```python
from build123d import *

# Parameters (mm, degrees)
SKETCH1_W                  = 37.6666666
SKETCH1_H                  = 45
BOSS_EXTRUDE1_DEPTH        = 12.8
SKETCH2_W                  = 10
SKETCH2_H                  = 34
CUT_EXTRUDE1_DEPTH         = 61.063447893
CUT_EXTRUDE2_DEPTH         = 6.4
CUT_EXTRUDE3_DEPTH         = 61.063447893
CUT_EXTRUDE4_DEPTH         = 6.4
CUT_EXTRUDE5_DEPTH         = 61.063447893
F_2_7_2_7_DIAMETER_HOLE1_D = 2.7
FILLET1_R                  = 2


with BuildPart() as part:
    # Sketch1 → Boss-Extrude1 (new body)
    with BuildSketch(Plane(origin=(0, 0, 0), x_dir=(0, 0, -1), z_dir=(1, 0, 0))):
        with Locations((-18.8333333, 22.5)):
            Rectangle(SKETCH1_W, SKETCH1_H)
    extrude(amount=-BOSS_EXTRUDE1_DEPTH)

    # Sketch2 → Cut-Extrude1 (cut, through all)
    with BuildSketch(Plane.ZY.offset(12.8)):
        with Locations((32.6666666, 28)):
            Rectangle(SKETCH2_W, SKETCH2_H)
    extrude(amount=-CUT_EXTRUDE1_DEPTH, mode=Mode.SUBTRACT)

    # Sketch3 → Cut-Extrude2 (cut)
    with BuildSketch(Plane(origin=(0, 0, 0), x_dir=(0, 0, -1), z_dir=(1, 0, 0))):
        with BuildLine():
            Line((-23.4933333, 39), (-23.4933333, 19))
            ThreePointArc((-23.4933333, 19), (-19.9933333, 15.5), (-16.4933333, 19))
            Line((-16.4933333, 19), (-16.4933333, 39))
            ThreePointArc((-16.4933333, 39), (-19.9933333, 42.5), (-23.4933333, 39))
        make_face()
    extrude(amount=-CUT_EXTRUDE2_DEPTH, mode=Mode.SUBTRACT)

    # Sketch4 → Cut-Extrude3 (cut, through all)
    with BuildSketch(Plane.ZY.offset(12.8)):
        with BuildLine():
            Line((21.4933333, 19), (21.4933333, 39))
            ThreePointArc((21.4933333, 39), (19.9933333, 40.5), (18.4933333, 39))
            Line((18.4933333, 39), (18.4933333, 19))
            ThreePointArc((18.4933333, 19), (19.9933333, 17.500288491), (21.4933333, 19))
        make_face()
    extrude(amount=-CUT_EXTRUDE3_DEPTH, mode=Mode.SUBTRACT)

    # Sketch5 → Cut-Extrude4 (cut)
    with BuildSketch(Plane(origin=(0, 0, 0), x_dir=(0, 0, -1), z_dir=(1, 0, 0))):
        with BuildLine():
            Line((-11.16, 39), (-11.16, 19))
            ThreePointArc((-11.16, 19), (-7.66, 15.5), (-4.16, 19))
            Line((-4.16, 19), (-4.16, 39))
            ThreePointArc((-4.16, 39), (-7.66, 42.5), (-11.16, 39))
        make_face()
    extrude(amount=-CUT_EXTRUDE4_DEPTH, mode=Mode.SUBTRACT)

    # Sketch6 → Cut-Extrude5 (cut, through all)
    with BuildSketch(Plane.ZY.offset(12.8)):
        with BuildLine():
            Line((6.16, 39), (6.16, 19))
            add(Edge.make_bspline(
                [(6.16, 19), (6.16, 18.832340191), (6.188940738, 18.662362459), (6.244463512, 18.504163113), (6.299983926, 18.345970491), (6.383577698, 18.195200889), (6.488243805, 18.06423361), (6.593105783, 17.93302124), (6.722000277, 17.818058166), (6.864319793, 17.728851239), (7.006949165, 17.639450093), (7.167029387, 17.573470631), (7.331255049, 17.536516135), (7.494915324, 17.499688864), (7.667199859, 17.490652088), (7.833819766, 17.510113335), (8.000323921, 17.529561063), (8.165758477, 17.578061145), (8.316432476, 17.651540351), (8.467050084, 17.724992056), (8.60707111, 17.825389016), (8.725036325, 17.944405925), (8.843438847, 18.063864039), (8.942888294, 18.205385466), (9.015071831, 18.357302993), (9.087259254, 18.5092287), (9.134141581, 18.67576982), (9.151759986, 18.843048139), (9.157247483, 18.895149292), (9.16, 18.947610662), (9.16, 19)],
                knots=[0, 0, 0, 0, 0.000502979, 0.000502979, 0.000502979, 0.001005909, 0.001005909, 0.001005909, 0.001509785, 0.001509785, 0.001509785, 0.002014828, 0.002014828, 0.002014828, 0.002518084, 0.002518084, 0.002518084, 0.003020994, 0.003020994, 0.003020994, 0.00352367, 0.00352367, 0.00352367, 0.004028264, 0.004028264, 0.004028264, 0.004532927, 0.004532927, 0.004532927, 0.004688075, 0.004688075, 0.004688075, 0.004688075], degree=3))
            Line((9.16, 19), (9.16, 39))
            add(Edge.make_bspline(
                [(9.16, 39), (9.16, 39.167659809), (9.131059262, 39.337637541), (9.075536488, 39.495836887), (9.020016074, 39.654029509), (8.936422302, 39.804799111), (8.831756195, 39.93576639), (8.726894217, 40.06697876), (8.597999723, 40.181941834), (8.455680207, 40.271148761), (8.313050835, 40.360549907), (8.152970613, 40.426529369), (7.988744951, 40.463483865), (7.825084676, 40.500311136), (7.652800141, 40.509347912), (7.486180234, 40.489886665), (7.319676079, 40.470438937), (7.154241523, 40.421938855), (7.003567524, 40.348459649), (6.852949916, 40.275007944), (6.71292889, 40.174610984), (6.594963675, 40.055594075), (6.476561153, 39.936135961), (6.377111706, 39.794614534), (6.304928169, 39.642697007), (6.232740746, 39.4907713), (6.185858419, 39.32423018), (6.168240014, 39.156951861), (6.162752517, 39.104850708), (6.16, 39.052389338), (6.16, 39)],
                knots=[0, 0, 0, 0, 0.000502979, 0.000502979, 0.000502979, 0.001005909, 0.001005909, 0.001005909, 0.001509785, 0.001509785, 0.001509785, 0.002014828, 0.002014828, 0.002014828, 0.002518084, 0.002518084, 0.002518084, 0.003020994, 0.003020994, 0.003020994, 0.00352367, 0.00352367, 0.00352367, 0.004028264, 0.004028264, 0.004028264, 0.004532927, 0.004532927, 0.004532927, 0.004688075, 0.004688075, 0.004688075, 0.004688075], degree=3))
        make_face()
    extrude(amount=-CUT_EXTRUDE5_DEPTH, mode=Mode.SUBTRACT)

    # Ø2.7 (2.7) Diameter Hole1 (through all)
    with Locations(Plane(origin=(0, 0, 0), x_dir=(0, 0, -1), z_dir=(1, 0, 0))):
        with Locations((-22.9666666, 3.3), (-32.4666666, 3.3)):
            Hole(F_2_7_2_7_DIAMETER_HOLE1_D / 2)

    # Fillet1
    fillet1_edges = [part.edges().sort_by_distance(p)[0] for p in [
        (-6.4, 45, 27.6666666),
        (-6.4, 11, 37.6666666),
        (-6.4, 11, 27.6666666),
        (-6.4, 0, 37.6666666),
        (-6.4, 45, 0),
        (-6.4, 0, 0),
    ]]
    fillet(fillet1_edges, radius=FILLET1_R)


solid = part.part
```
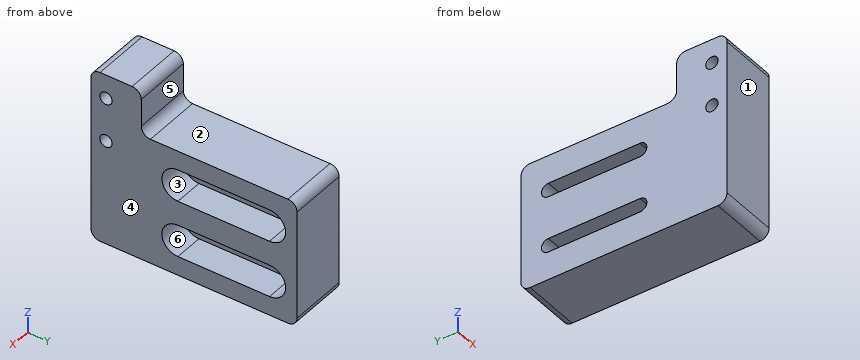
Work out the finished part from the listing and answer in its coordinate system (mm). Face numbers are marked on the shaded views. A direction names the side the tool comes from. Give positions to 0.01 mm unless a question says otherwise; leave off trailing zeros. Write each loop counter-clockwise with the first axis right and the second up, starting at its lowest first coordinate (ties: lowest second). Pieces come first, ordered by that corner, then holes.
(1) Flat-ended cylindrical pins translate along their axes: pin 1 Ø1.9 at (x, y) = (-11, 33) entering from +Z; pin 2 Ø2.5 at (y, z) = (3.3, 22.97) entering from +X; pin 3 Ø7.5 at (y, z) = (30, 8) entering from +X; pin 4 Ø3 at (x, z) = (-4, 32) entering from +Y. Find the tip coordinate at first contact, or state that the pin passes through.
Final values:
pin 1: stops at z = 27.67
pin 2: passes through
pin 3: stops at x = 0
pin 4: stops at y = 11
(2) Straight lines are drawn through the part: line 1 (Z direction, x = -0.75, y = 26); line 2 (Z direction, x = -9.25, y = 20.5); line 3 (Z direction, x = -7.5, y = 41). For each, find the intervals that lie inside material, in ascending order.
Final values:
line 1: z = 0 to 4.16, 11.16 to 16.49, 23.49 to 27.67
line 2: z = 0 to 6.16, 9.16 to 18.49, 21.49 to 27.67
line 3: z = 0 to 27.67
(3) The part is cut by section A-A on y = 3.3. Write down the section's boundary in (x, z).
Final values:
outline: (-12.8, 0) - (0, 0) - (0, 21.62) - (-12.8, 21.62) - close; (-12.8, 24.32) - (0, 24.32) - (0, 31.12) - (-12.8, 31.12) - close; (-12.8, 33.82) - (0, 33.82) - (0, 37.67) - (-12.8, 37.67) - close
(4) The mould has two halves that part along Z. Classify the marked faces 1, 2 and 3: pulls with the +Z half, pulls with the -Z half, needs draft (parallel to the pull), parting line crosses it, or undercut.
Final values:
face 1: needs draft
face 2: pulls with the +Z half
face 3: undercut
(5) The part is cut by section B-B on x = -7. Count the separate pieces of the cut face and the enclosed holes in it, plus the area to 3 significant figures.
Final values:
separate pieces: 1
enclosed holes: 4
area: 1,210 mm2
(6) The part is cut by section C-C on y = 37.5. Write down the section's boundary in (x, z), plus the area to 3 significant figures.
Final values:
outline: (-12.8, 0) - (0, 0) - (0, 4.16) - (-6.4, 4.16) - (-6.4, 6.16) - (-12.8, 6.16) - close; (-12.8, 9.16) - (-6.4, 9.16) - (-6.4, 11.16) - (0, 11.16) - (0, 16.49) - (-6.4, 16.49) - (-6.4, 18.49) - (-12.8, 18.49) - close; (-12.8, 21.49) - (-6.4, 21.49) - (-6.4, 23.49) - (0, 23.49) - (0, 27.67) - (-12.8, 27.67) - close
area: 226 mm2
(7) Which of the six approach directions +Z, -Z, +X, -X, +Y, -Y give full straight-line access (tool end or side, diameter ignored) to the marked faces 4, 5 and 6?
Final values:
face 4: +Z, -Z, +X, +Y, -Y
face 5: +Z, +X, -X, +Y
face 6: +X
(8) The part is cut by section D-D on y = 16. Write down the section's boundary in (x, z).
Final values:
outline: (-12.8, 0) - (0, 0) - (0, 5.86) - (-6.4, 5.86) - (-6.4, 9.46) - (0, 9.46) - (0, 18.19) - (-6.4, 18.19) - (-6.4, 21.8) - (0, 21.8) - (0, 27.67) - (-12.8, 27.67) - close
